Print and shaded views of the part. All mm, measured from the part's lowest x, y and z. A direction names the side the tool comes from. Give positions to 0.01 mm unless a question says otherwise; leave off trailing zeros. Loops run counter-clockwise (first coordinate to the right, second up) from the corner with the lowest first, then second, coordinate; pieces in that order, holes last. Notation, with made-up numbers: (46.25, 7.5) -> (51.25, 7.5) arc R35 ccw to (51.25, 45.5) -> close; hole circle Ø10 at (-2, 78.5). An arc over 180 degrees is marked (long way). Answer as a JSON object with one key per item and string values. Group by question number.
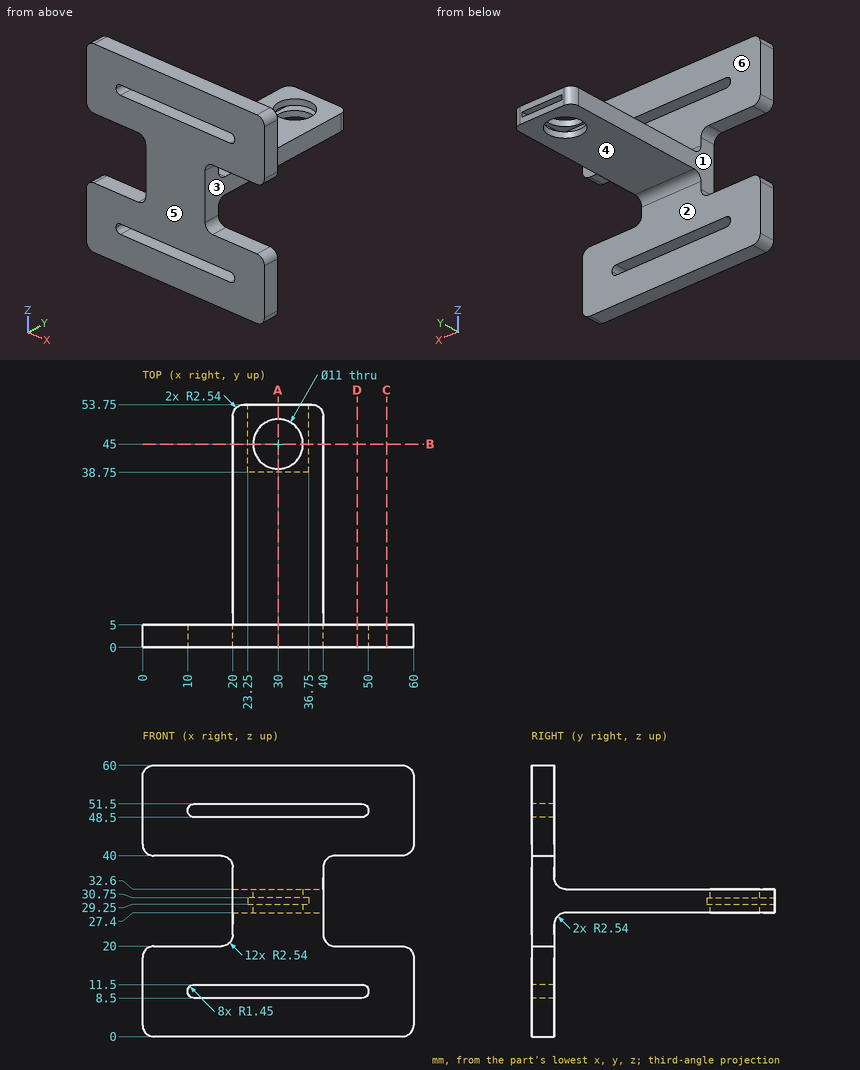
(1) 3-axis set-ups, long thin cutter, end or side, ignore diameter. For the marked faces 5 and 6: which of +Z, -Z, +X, -X, +Y, -Y reach the whole face in a straight line?
(2) Saw through at C-C on x = 54. List the corners of the cut face in (y, z), plus the area to 3 significant figures.
(3) Saw through at B-B on y = 45. List the corners of the cut face in (x, z).
(4) Saw through at D-D on x = 47.5. List the corners of the cut face in (y, z).
(5) Probe line 1 along Z through (x, y) = (14, 4.5); line 2 along Y through (x, z) = (30, 31); line 3 along Z through (x, y) = (20.5, 12). List the from-to ranges inside material, lowest first. Write a range as [from, to].
(6) Pull direction Z, two halves, no side cores. Call the marked faces 1, 2, 3 and 4: pulls with the +Z half, pulls with the -Z half, needs draft (parallel to the pull), parting line crosses it, or undercut.
(7) Saw through at A-A on x = 30. Give the number of separate pieces and of enclosed holes in the cut face, plus the area to 3 significant figures.
(8) Pin check, flat tips, straight feed: pin 1 (7.5 mm diameter, centred on x = 28, z = 44.5, fed in from +Y); pin 2 (5 mm diameter, centred on x = 41, y = 25.5, fed in from +Z); pin 3 (5 mm diameter, centred on x = 43.5, y = 40.5, fed in from +Z); pin 4 (7 mm diameter, centred on x = 33.5, y = 48.5, fed in from -Z). Stop position of each tip, or through.
Calculated:
{
 "1": {"face 5": "+Z, -Z, +X, -X, -Y", "face 6": "+Z, +X, -X, +Y"},
 "2": {"outline": "(0, 0) -> (5, 0) -> (5, 20) -> (0, 20) -> close; (0, 40) -> (5, 40) -> (5, 60) -> (0, 60) -> close", "area": "200 mm^2"},
 "3": {"outline": "(20, 27.4) -> (24.5, 27.4) -> (24.5, 29.25) -> (23.25, 29.25) -> (23.25, 30.75) -> (24.5, 30.75) -> (24.5, 32.6) -> (20, 32.6) -> close; (35.5, 27.4) -> (40, 27.4) -> (40, 32.6) -> (35.5, 32.6) -> (35.5, 30.75) -> (36.75, 30.75) -> (36.75, 29.25) -> (35.5, 29.25) -> close"},
 "4": {"outline": "(0, 0) -> (5, 0) -> (5, 8.5) -> (0, 8.5) -> close; (0, 11.5) -> (5, 11.5) -> (5, 20) -> (0, 20) -> close; (0, 40) -> (5, 40) -> (5, 48.5) -> (0, 48.5) -> close; (0, 51.5) -> (5, 51.5) -> (5, 60) -> (0, 60) -> close"},
 "5": {"line 1": "z = [0, 8.5], [11.5, 20], [40, 48.5], [51.5, 60]", "line 2": "y = [0, 39.5], [50.5, 53.75]", "line 3": "z = [27.4, 32.6]"},
 "6": {"face 1": "undercut", "face 2": "needs draft", "face 3": "undercut", "face 4": "pulls with the -Z half"},
 "7": {"separate pieces": "5", "enclosed holes": "0", "area": "463 mm^2"},
 "8": {"pin 1": "stops at y = 5", "pin 2": "stops at z = 32.6", "pin 3": "passes through", "pin 4": "stops at z = 27.4"}
}
